Input: part model. Units: mm. Frame: model coordinates. Face numbers are marked on the shaded views. Round coordinates to 2 decimals unless told otherwise and drop trailing zeros. Loops run counter-clockwise (first coordinate to the right, second up) from the corner with the lowest first, then second, coordinate; pieces in that order, holes last. Notation, with made-up numbers: (-36.75, 50.25) -> (5.25, 50.25) arc R22 cw to (5.25, 82.25) -> close; hole circle Ø6 at (16, 26). An arc over 180 degrees is marked (long way). Answer in a Markdown table with one row per item. Add a question column.
Q1. Section D-D, the plane z = 4.75. Output: boundary loops of the cut face in (x, y), and give its area (3 significant figures).
Q2. Section C-C, the plane y = -5.5. Output: boundary loops of the cut face in (x, z), and give its area (3 significant figures).
Q3. Section B-B, the plane z = 0. Output: boundary loops of the cut face in (x, y), and give its area (3 significant figures).
Q4. Ray query, L1, parallel to Z at x = 0, y = -4.6; L2, parallel to X at y = -0.25, z = -1; L3, parallel to X at y = -0.9, z = 1.5. Return the intervals inside material, ascending. Write a range as from..to.
Q5. Mould query, pull axis X, two halves, no side actions, for the marked faces 1, 2 and 3. Classes: pulls with the +X half, pulls with the -X half, needs draft (parallel to the pull), parting line crosses it, or undercut.
Q6. Section A-A, the plane x = 0. Output: boundary loops of the cut face in (y, z).
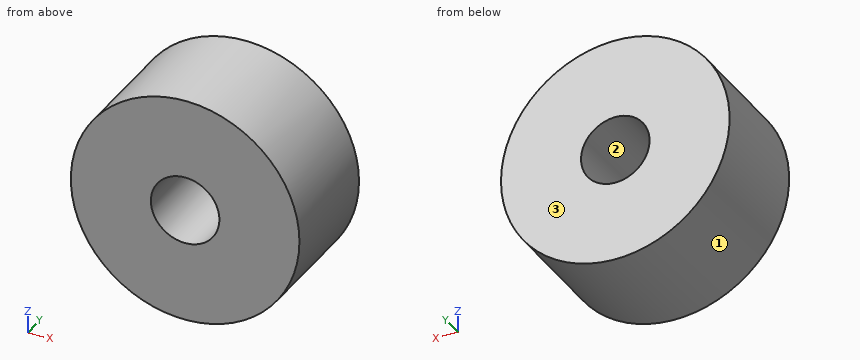
```python
from build123d import *

# Parameters (mm, degrees)
CYLINDER011030_R     = 1.8
CYLINDER011030_DEPTH = 20
CYLINDER011031_R     = 6
CYLINDER011031_DEPTH = 6


with BuildPart() as belt_attach_bolt_hole:
    # Cylinder011030 → Cylinder011030 (new body)
    with BuildSketch(Plane.XZ):
        Circle(CYLINDER011030_R)
    extrude(amount=CYLINDER011030_DEPTH)


with BuildPart() as belt_horizontal_attach_washer_cut:
    # Cylinder011031 → Cylinder011031 (new body)
    with BuildSketch(Plane.XZ):
        Circle(CYLINDER011031_R)
    extrude(amount=CYLINDER011031_DEPTH)

    # Cut023015009021: cut belt attach bolt hole
    add(belt_attach_bolt_hole.part, mode=Mode.SUBTRACT)


solid = belt_horizontal_attach_washer_cut.part
```
Answer block:
| question | item | result |
|---|---|---|
| 1 | outline | (-3.67, -6) -> (3.67, -6) -> (3.67, 0) -> (-3.67, 0) -> close |
| 1 | area | 44.0 mm^2 |
| 2 | outline | circle Ø12 at (0, 0); hole circle Ø3.6 at (0, 0) |
| 2 | area | 103 mm^2 |
| 3 | outline | (-6, -6) -> (-1.8, -6) -> (-1.8, 0) -> (-6, 0) -> close; (1.8, -6) -> (6, -6) -> (6, 0) -> (1.8, 0) -> close |
| 3 | area | 50.4 mm^2 |
| 4 | L1 | -6..-1.8, 1.8..6 |
| 4 | L2 | -5.92..-1.5, 1.5..5.92 |
| 4 | L3 | -5.81..-0.99, 0.99..5.81 |
| 5 | face 1 | parting line crosses it |
| 5 | face 2 | undercut |
| 5 | face 3 | needs draft |
| 6 | outline | (-6, -6) -> (0, -6) -> (0, -1.8) -> (-6, -1.8) -> close; (-6, 1.8) -> (0, 1.8) -> (0, 6) -> (-6, 6) -> close |
